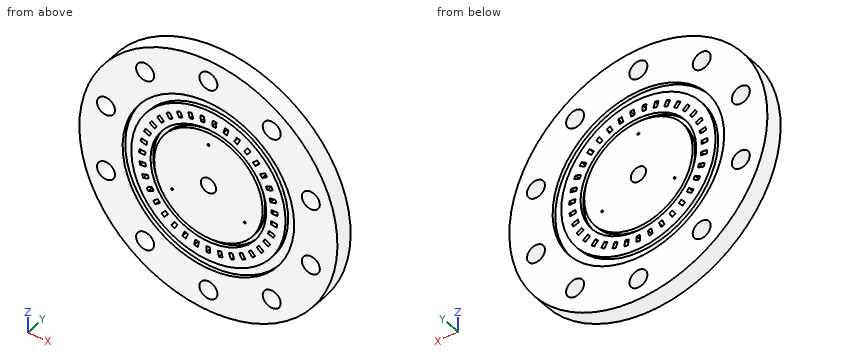
from build123d import *

# Parameters (mm, degrees)
SKETCH1_R                       = 107.826846
SKETCH1_R_2                     = 7.5
SKETCH1_R_3                     = 6.35
FACEPLATE_EXTRUSION_DEPTH       = 15
REGEN_CHANNELS_W                = 3
REGEN_CHANNELS_H                = 5
REGEN_CHANNEL_DEPTH             = 154.226164334
REGEN_CHANNELS_REVOLVE_COUNT    = 35
SKETCH30_R                      = 71.686846
SKETCH30_R_2                    = 64.447846
INTERFACING_O_RING_SLOT_1_DEPTH = 3
INTERFACING_START               = -3
SKETCH32_R                      = 71.687
SKETCH32_R_2                    = 64.447846
INTERFACING_O_RING_SLOT_2_DEPTH = 3
SKETCH33_R                      = 48.33
SKETCH33_R_2                    = 45.33
MANIFOLD_O_RING_SLOT_1_DEPTH    = 3
MANIFOLD_START                  = -3
SKETCH34_R                      = 48.33
SKETCH34_R_2                    = 45.33
MANIFOLD_O_RING_SLOT_2_DEPTH    = 3
SKETCH35_R                      = 0.8262
FUEL_BYPASS_CHANNELS_DEPTH      = 154.226164334


with BuildPart() as part:
    # Sketch1 → Faceplate Extrusion (new body)
    with BuildSketch(Plane(origin=(0, 0, 0), x_dir=(1, 0, 0), z_dir=(0, 1, 0))):
        with Locations(Location((0, 0, 0), (0, 0, 270))):
            Circle(SKETCH1_R)
        with Locations(Location((0, 90, 0), (0, 0, 270))):
            Circle(SKETCH1_R_2, mode=Mode.SUBTRACT)
        with Locations(Location((52.900672706, 72.811529494, 0), (0, 0, 270))):
            Circle(SKETCH1_R_2, mode=Mode.SUBTRACT)
        with Locations(Location((85.595086467, 27.811529494, 0), (0, 0, 270))):
            Circle(SKETCH1_R_2, mode=Mode.SUBTRACT)
        with Locations(Location((85.595086467, -27.811529494, 0), (0, 0, 270))):
            Circle(SKETCH1_R_2, mode=Mode.SUBTRACT)
        with Locations(Location((52.900672706, -72.811529494, 0), (0, 0, 270))):
            Circle(SKETCH1_R_2, mode=Mode.SUBTRACT)
        with Locations(Location((0, -90, 0), (0, 0, 270))):
            Circle(SKETCH1_R_2, mode=Mode.SUBTRACT)
        with Locations(Location((-52.900672706, -72.811529494, 0), (0, 0, 270))):
            Circle(SKETCH1_R_2, mode=Mode.SUBTRACT)
        with Locations(Location((-85.595086467, -27.811529494, 0), (0, 0, 270))):
            Circle(SKETCH1_R_2, mode=Mode.SUBTRACT)
        with Locations(Location((-85.595086467, 27.811529494, 0), (0, 0, 270))):
            Circle(SKETCH1_R_2, mode=Mode.SUBTRACT)
        with Locations(Location((-52.900672706, 72.811529494, 0), (0, 0, 270))):
            Circle(SKETCH1_R_2, mode=Mode.SUBTRACT)
        with Locations(Location((0, 0, 0), (0, 0, 270))):
            Circle(SKETCH1_R_3, mode=Mode.SUBTRACT)
    extrude(amount=FACEPLATE_EXTRUSION_DEPTH)

    # Regen Channels → Regen Channel (cut, through all)
    with BuildSketch(Plane(origin=(0, 15, 0), x_dir=(1, 0, 0), z_dir=(0, 1, 0))):
        with Locations((0, 55.326846)):
            Rectangle(REGEN_CHANNELS_W, REGEN_CHANNELS_H)
    regen_channel = extrude(amount=-REGEN_CHANNEL_DEPTH, mode=Mode.SUBTRACT)

    # Regen Channels Revolve: Regen Channel ×35 about axis
    regen_channels_revolve_axis = Axis((0, 0, 0), (0, 1, 0))
    for i in range(1, REGEN_CHANNELS_REVOLVE_COUNT):
        add(regen_channel.rotate(regen_channels_revolve_axis, i * 360 / REGEN_CHANNELS_REVOLVE_COUNT), mode=Mode.SUBTRACT)

    # Sketch30 → Interfacing O-Ring Slot 1 (cut)
    with BuildSketch(Plane.XZ):
        with Locations(Location((0, 0, 0), (0, 0, 270))):
            Circle(SKETCH30_R)
        with Locations(Location((0, 0, 0), (0, 0, 270))):
            Circle(SKETCH30_R_2, mode=Mode.SUBTRACT)
    extrude(amount=-INTERFACING_O_RING_SLOT_1_DEPTH, mode=Mode.SUBTRACT)

    # Sketch32 → Interfacing O-Ring Slot 2 (cut)
    with BuildSketch(Plane(origin=(0, 15, 0), x_dir=(1, 0, 0), z_dir=(0, 1, 0)).offset(INTERFACING_START)):
        with Locations(Location((0, 0, 0), (0, 0, 270))):
            Circle(SKETCH32_R)
        with Locations(Location((0, 0, 0), (0, 0, 90))):
            Circle(SKETCH32_R_2, mode=Mode.SUBTRACT)
    extrude(amount=INTERFACING_O_RING_SLOT_2_DEPTH, mode=Mode.SUBTRACT)

    # Sketch33 → Manifold O-Ring Slot 1 (cut)
    with BuildSketch(Plane(origin=(0, 15, 0), x_dir=(1, 0, 0), z_dir=(0, 1, 0))):
        with Locations(Location((0, 0, 0), (0, 0, 270))):
            Circle(SKETCH33_R)
        with Locations(Location((0, 0, 0), (0, 0, 270))):
            Circle(SKETCH33_R_2, mode=Mode.SUBTRACT)
    extrude(amount=-MANIFOLD_O_RING_SLOT_1_DEPTH, mode=Mode.SUBTRACT)

    # Sketch34 → Manifold O-Ring Slot 2 (cut)
    with BuildSketch(Plane.XZ.offset(MANIFOLD_START)):
        with Locations(Location((0, 0, 0), (0, 0, 90))):
            Circle(SKETCH34_R)
        with Locations(Location((0, 0, 0), (0, 0, 90))):
            Circle(SKETCH34_R_2, mode=Mode.SUBTRACT)
    extrude(amount=MANIFOLD_O_RING_SLOT_2_DEPTH, mode=Mode.SUBTRACT)

    # Sketch35 → Fuel Bypass Channels (cut, through all)
    with BuildSketch(Plane.XZ):
        with Locations(Location((0, 35, 0), (0, 0, 270))):
            Circle(SKETCH35_R)
        with Locations(Location((30.310889132, -17.5, 0), (0, 0, 270))):
            Circle(SKETCH35_R)
        with Locations(Location((-30.310889132, -17.5, 0), (0, 0, 270))):
            Circle(SKETCH35_R)
    extrude(amount=-FUEL_BYPASS_CHANNELS_DEPTH, mode=Mode.SUBTRACT)


solid = part.part
Design review of the part built by this model. Coordinates are the model's own, in mm. Give positions to 0.01 mm unless a question says otherwise; leave off trailing zeros.
1. For pin 1 Ø3 at (x, y) = (-73, 4.5) entering from -Z; pin 2 Ø10 at (x, z) = (0, 0) entering from -Y; pin 3 Ø6 at (y, z) = (12, 42.5) entering from +X; pin 4 Ø6 at (y, z) = (6.5, 18) entering from +X, all flat-tipped, find the tip position at first contact; note any pin that passes through.
Solution:
pin 1: stops at z = -80.71
pin 2: passes through
pin 3: stops at x = 100.33
pin 4: stops at x = 106.78
2. To check wall thickness, follow L1, parallel to Z at x = -59, y = 9.5; L2, parallel to X at y = 9.5, z = -0.5; L3, parallel to X at y = 2.25, z = 0. State the ranges of each line that lie inside material, in increasing order.
Solution:
L1: z = -90.25 to -77.18, -68.45 to 68.45, 77.18 to 90.25
L2: x = -107.83 to -6.33, 6.33 to 107.83
L3: x = -107.83 to -71.69, -64.45 to -48.33, -45.33 to -6.35, 6.35 to 45.33, 48.33 to 64.45, 71.69 to 107.83
3. Add section A-A, the plane y = 9.75. State how many separate pieces and enclosed holes the cut face has, then the cut area to 3 significant figures.
Solution:
separate pieces: 1
enclosed holes: 49
area: 34,100 mm2
